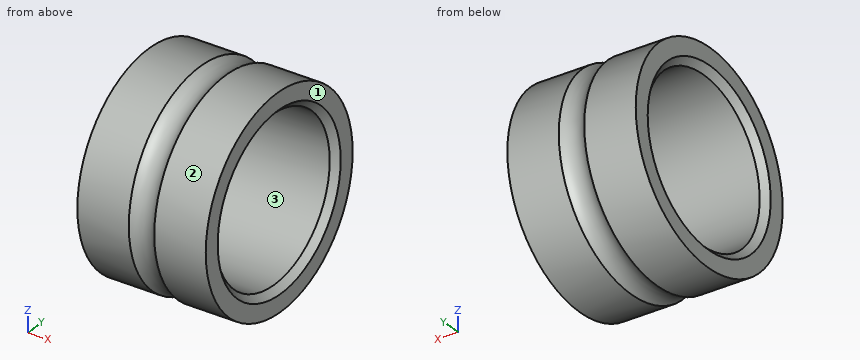
Autodesk Inventor part; units mm, degrees
ref_plane "center_or_XY" through (0, 0, 0) normal (1, 0, 0) x (0, 0, -1)
ref_plane "center_or_YZ" through (0, 0, 0) normal (0, 0, -1) x (0, 1, 0)
ref_plane "center_or_ZX" through (0, 0, 0) normal (0, 1, 0) x (1, 0, 0)
sketch "Sketch_2" plane through (0, 0, 0) normal (0, 0, 1) x (1, 0, 0)
  line L0 (4, 0) -> (0, 0)
  line L1 (0, 3.225) -> (0, 2.7)
  line L2 (0, 2.7) -> (0.2, 2.5)
  line L3 (0.2, 2.5) -> (3.8, 2.5)
  line L4 (3.8, 2.5) -> (4, 2.7)
  line L5 (4, 2.7) -> (4, 3.225)
  line L6 (4, 3.225) -> (2.3969, 3.225)
  arc A0 (1.6031, 3.225) -> (2.3969, 3.225) centre (2, 3.675) ccw
  line L7 (1.6031, 3.225) -> (0, 3.225)
revolve "Revolution1" add sketch "Sketch_2" angle 360 about axis through (4, 0, 0) along (1, 0, 0)
ref_plane "center_or_XY" through (0, 0, 0) normal (1, 0, 0) x (0, 0, -1)
ref_plane "center_or_YZ" through (0, 0, 0) normal (0, 0, -1) x (0, 1, 0)
ref_plane "center_or_ZX" through (0, 0, 0) normal (0, 1, 0) x (1, 0, 0)
properties part number "WML5010ZZ Inner ring"
Source: CAD feature listing. Evaluate the final solid. Frame: model axes, mm. Face numbers are marked on the shaded views. Round coordinates to 2 decimals unless told otherwise and drop trailing zeros. Write each loop counter-clockwise with the first axis right and the second up, starting at its lowest first coordinate (ties: lowest second). Pieces come first, ordered by that corner, then holes. Notation, with made-up numbers: (53, 50) - (80, 50) arc R16 cw to (80, 68) - close; hole circle Ø3 at (28, 33.5). An arc over 180 degrees is marked (long way). Use CSV: the item, a comma, the result in double quotes. Start each with the question number.
(1) First-contact query: pin 1 Ø3 at (y, z) = (0, 0) entering from -X. Flat tip, straight axial feed; report the tip coordinate or a pass-through.
(2) Cut plane D-D, the plane x = 1.75. Return loops of the section in (y, z).
(3) Cut plane A-A, the plane z = 0. Return loops of the section in (x, y) (3 decimals), and give its area (3 significant figures).
(4) Material intervals for probe 1 along Z at (x, y) = (3.1, 0) (3 decimals); probe 2 along Z at (x, y) = (0.8, -2.25); probe 3 along Y at (x, z) = (3.5, -2), sorted ascending. Write a range as [from, to].
(5) Mould query, pull axis Z, two halves, no side actions, for the marked faces 1, 2 and 3. Classes: pulls with the +Z half, pulls with the -Z half, needs draft (parallel to the pull), parting line crosses it, or undercut.
(6) Cut plane C-C, the plane x = 3.1. Return loops of the section in (y, z) (3 decimals).
Geometry says:
1,pin 1,"through"
2,outline,"circle Ø6.26 at (0, 0); hole circle Ø5 at (0, 0)"
3,outline,"(0, -3.225) - (1.603, -3.225) arc R0.6 cw to (2.397, -3.225) - (4, -3.225) - (4, -2.7) - (3.8, -2.5) - (0.2, -2.5) - (0, -2.7) - close; (0, 2.7) - (0.2, 2.5) - (3.8, 2.5) - (4, 2.7) - (4, 3.225) - (2.397, 3.225) arc R0.6 cw to (1.603, 3.225) - (0, 3.225) - close"
3,area,"5.56 mm²"
4,probe 1,"[-3.225, -2.5], [2.5, 3.225]"
4,probe 2,"[-2.31, -1.09], [1.09, 2.31]"
4,probe 3,"[-2.53, -1.5], [1.5, 2.53]"
5,face 1,"needs draft"
5,face 2,"parting line crosses it"
5,face 3,"undercut"
6,outline,"circle Ø6.45 at (0, 0); hole circle Ø5 at (0, 0)"
